from build123d import *

# Parameters (mm, degrees)
SKETCH1_W           = 177.2
SKETCH1_H           = 161.6
BOSS_EXTRUDE1_DEPTH = 10


with BuildPart() as part:
    # Sketch1 → Boss-Extrude1 (new body)
    with BuildSketch(Plane(origin=(0, 0, 0), x_dir=(1, 0, 0), z_dir=(0, 1, 0))):
        with Locations((88.6, 80.8)):
            Rectangle(SKETCH1_W, SKETCH1_H)
        Polygon((5, 36.112698372), (5, 12.687301628), (12.687301628, 5), (36.112698372, 5), (43.8, 12.687301628), (43.8, 36.112698372), (36.112698372, 43.8), (12.687301628, 43.8), align=None, mode=Mode.SUBTRACT)
        Polygon((55.487301628, 43.8), (47.8, 36.112698372), (47.8, 12.687301628), (55.487301628, 5), (78.912698372, 5), (86.6, 12.687301628), (86.6, 36.112698372), (78.912698372, 43.8), align=None, mode=Mode.SUBTRACT)
        Polygon((98.287301628, 43.8), (90.6, 36.112698372), (90.6, 12.687301628), (98.287301628, 5), (121.712698372, 5), (129.4, 12.687301628), (129.4, 36.112698372), (121.712698372, 43.8), align=None, mode=Mode.SUBTRACT)
        Polygon((141.087301628, 43.8), (133.4, 36.112698372), (133.4, 12.687301628), (141.087301628, 5), (164.512698372, 5), (172.2, 12.687301628), (172.2, 36.112698372), (164.512698372, 43.8), align=None, mode=Mode.SUBTRACT)
        Polygon((55.487301628, 86.6), (47.8, 78.912698372), (47.8, 55.487301628), (55.487301628, 47.8), (78.912698372, 47.8), (86.6, 55.487301628), (86.6, 78.912698372), (78.912698372, 86.6), align=None, mode=Mode.SUBTRACT)
        Polygon((98.287301628, 86.6), (90.6, 78.912698372), (90.6, 55.487301628), (98.287301628, 47.8), (121.712698372, 47.8), (129.4, 55.487301628), (129.4, 78.912698372), (121.712698372, 86.6), align=None, mode=Mode.SUBTRACT)
        Polygon((141.087301628, 86.6), (133.4, 78.912698372), (133.4, 55.487301628), (141.087301628, 47.8), (164.512698372, 47.8), (172.2, 55.487301628), (172.2, 78.912698372), (164.512698372, 86.6), align=None, mode=Mode.SUBTRACT)
        Polygon((12.687301628, 86.6), (5, 78.912698372), (5, 55.487301628), (12.687301628, 47.8), (36.112698372, 47.8), (43.8, 55.487301628), (43.8, 78.912698372), (36.112698372, 86.6), align=None, mode=Mode.SUBTRACT)
        Polygon((9.4, 113.873863607), (9.4, 99.326136393), (17.126136393, 91.6), (31.673863607, 91.6), (39.4, 99.326136393), (39.4, 113.873863607), (31.673863607, 121.6), (17.126136393, 121.6), align=None, mode=Mode.SUBTRACT)
        Polygon((52.2, 113.873863607), (52.2, 99.326136393), (59.926136393, 91.6), (74.473863607, 91.6), (82.2, 99.326136393), (82.2, 113.873863607), (74.473863607, 121.6), (59.926136393, 121.6), align=None, mode=Mode.SUBTRACT)
        Polygon((95, 113.873863607), (95, 99.326136393), (102.726136393, 91.6), (117.273863607, 91.6), (125, 99.326136393), (125, 113.873863607), (117.273863607, 121.6), (102.726136393, 121.6), align=None, mode=Mode.SUBTRACT)
        Polygon((137.8, 113.873863607), (137.8, 99.326136393), (145.526136393, 91.6), (160.073863607, 91.6), (167.8, 99.326136393), (167.8, 113.873863607), (160.073863607, 121.6), (145.526136393, 121.6), align=None, mode=Mode.SUBTRACT)
        Polygon((52.2, 148.873863607), (52.2, 134.326136393), (59.926136393, 126.6), (74.473863607, 126.6), (82.2, 134.326136393), (82.2, 148.873863607), (74.473863607, 156.6), (59.926136393, 156.6), align=None, mode=Mode.SUBTRACT)
        Polygon((95, 148.873863607), (95, 134.326136393), (102.726136393, 126.6), (117.273863607, 126.6), (125, 134.326136393), (125, 148.873863607), (117.273863607, 156.6), (102.726136393, 156.6), align=None, mode=Mode.SUBTRACT)
        Polygon((137.8, 148.873863607), (137.8, 134.326136393), (145.526136393, 126.6), (160.073863607, 126.6), (167.8, 134.326136393), (167.8, 148.873863607), (160.073863607, 156.6), (145.526136393, 156.6), align=None, mode=Mode.SUBTRACT)
        Polygon((9.4, 148.873863607), (9.4, 134.326136393), (17.126136393, 126.6), (31.673863607, 126.6), (39.4, 134.326136393), (39.4, 148.873863607), (31.673863607, 156.6), (17.126136393, 156.6), align=None, mode=Mode.SUBTRACT)
    extrude(amount=BOSS_EXTRUDE1_DEPTH)


solid = part.part
Can you work these out from the model? Positions are in its coordinate system, mm. Give positions to 0.01 mm unless a question says otherwise; leave off trailing zeros. Write each loop counter-clockwise with the first axis right and the second up, starting at its lowest first coordinate (ties: lowest second). Pieces come first, ordered by that corner, then holes. Notation, with made-up numbers: M -38.5,-34 L 14.5,-34 A20 ccw 14.5,-20 Z; hole C 44,36 d8. An arc over 180 degrees is marked long. Answer in a Markdown table with one row per item. Add a question column.
Item 1: Imagine slicing it at B-B, the plane x = 69. Write out the boundary of the cut face in (y, z).
Item 2: Please list where these lines run through material, in increasing order: L1, parallel to X at y = 9.75, z = -73.5; L2, parallel to X at y = 1, z = -147; L3, parallel to Z at x = 147.5, y = 2.
Item 3: Imagine slicing it at C-C, the plane y = 4. State how many separate pieces and enclosed holes the cut face has, plus the area to 3 significant figures.
Item 4: Imagine slicing it at A-A, the plane z = -23. Write out the boundary of the cut face in (x, y).
Evaluation:
| question | item | result |
|---|---|---|
| 1 | outline | M 0,-161.6 L 10,-161.6 L 10,-156.6 L 0,-156.6 Z; M 0,-126.6 L 10,-126.6 L 10,-121.6 L 0,-121.6 Z; M 0,-91.6 L 10,-91.6 L 10,-86.6 L 0,-86.6 Z; M 0,-47.8 L 10,-47.8 L 10,-43.8 L 0,-43.8 Z; M 0,-5 L 10,-5 L 10,0 L 0,0 Z |
| 2 | L1 | x = 0 to 5, 43.8 to 47.8, 86.6 to 90.6, 129.4 to 133.4, 172.2 to 177.2 |
| 2 | L2 | x = 0 to 9.4, 39.4 to 52.2, 82.2 to 95, 125 to 137.8, 167.8 to 177.2 |
| 2 | L3 | z = -161.6 to -156.6, -126.6 to -121.6, -91.6 to -86.6, -47.8 to -43.8, -5 to 0 |
| 3 | separate pieces | 1 |
| 3 | enclosed holes | 16 |
| 3 | area | 11,300 mm² |
| 4 | outline | M 0,0 L 5,0 L 5,10 L 0,10 Z; M 43.8,0 L 47.8,0 L 47.8,10 L 43.8,10 Z; M 86.6,0 L 90.6,0 L 90.6,10 L 86.6,10 Z; M 129.4,0 L 133.4,0 L 133.4,10 L 129.4,10 Z; M 172.2,0 L 177.2,0 L 177.2,10 L 172.2,10 Z |
